Build history of the part. All positions in model axes, mm. A direction names the side the tool comes from. Coordinates: 2 decimals unless noted, no trailing zeros. Order: outer loops, then holes, each group sorted by start corner. A loop starts at its lowest first (then second) coordinate and runs counter-clockwise, first axis right, second up. Notation, with made-up numbers: (44, 35.25) - (96, 35.25) arc R23 cw to (96, 59.25) - close; hole circle Ø1 at (74.5, 42). An arc over 180 degrees is marked (long way). Write each question's results on one line, items separated by ' | '.
from build123d import *

# Parameters (mm, degrees)
BOSS_EXTRUDE1_DEPTH = 50
SKETCH2_R           = 2.8
CUT_EXTRUDE1_DEPTH  = 53.73966846


with BuildPart() as part:
    # Sketch1 → Boss-Extrude1 (new body)
    with BuildSketch(Plane.XY):
        with BuildLine():
            Line((-10.618380291, 0), (10.618380291, 0))
            Line((10.618380291, 0), (10.618380291, 6))
            ThreePointArc((10.618380291, 6), (7.305893165, 8.590308493), (3.395577503, 10.136820848))
            Line((3.395577503, 10.136820848), (3.395577503, 10.989327513))
            ThreePointArc((3.395577503, 10.989327513), (2.809791065, 12.403541075), (1.395577503, 12.989327513))
            Line((1.395577503, 12.989327513), (-1.395577503, 12.989327513))
            ThreePointArc((-1.395577503, 12.989327513), (-2.809791065, 12.403541075), (-3.395577503, 10.989327513))
            Line((-3.395577503, 10.989327513), (-3.395577503, 10.136820848))
            ThreePointArc((-3.395577503, 10.136820848), (-7.305893165, 8.590308493), (-10.618380291, 6))
            Line((-10.618380291, 6), (-10.618380291, 0))
        make_face()
    extrude(amount=-BOSS_EXTRUDE1_DEPTH)

    # Sketch2 → Cut-Extrude1 (cut, through all)
    with BuildSketch(Plane.XY):
        with Locations((-4, 4.84)):
            Circle(SKETCH2_R)
        with Locations((4, 4.84)):
            Circle(SKETCH2_R)
    extrude(amount=-CUT_EXTRUDE1_DEPTH, mode=Mode.SUBTRACT)


solid = part.part
1. Band-saw the part on C-C on x = -4. Give the cut face in (y, z), then the cut area to 3 significant figures.
Solved:
outline: (0, -50) - (2.04, -50) - (2.04, 0) - (0, 0) - close; (7.64, -50) - (9.98, -50) - (9.98, 0) - (7.64, 0) - close | area: 219 mm2
2. Band-saw the part on D-D on x = 5.5. Give the cut face in (y, z), then the cut area to 3 significant figures.
Solved:
outline: (0, -50) - (2.48, -50) - (2.48, 0) - (0, 0) - close; (7.2, -50) - (9.47, -50) - (9.47, 0) - (7.2, 0) - close | area: 237 mm2
3. Band-saw the part on A-A on y = 4.84. Give the cut face in (x, z), then the cut area to 3 significant figures.
Solved:
outline: (-10.62, -50) - (-6.8, -50) - (-6.8, 0) - (-10.62, 0) - close; (-1.2, -50) - (1.2, -50) - (1.2, 0) - (-1.2, 0) - close; (6.8, -50) - (10.62, -50) - (10.62, 0) - (6.8, 0) - close | area: 502 mm2
4. Probe line 1 (X direction, y = 2.5, z = -33.5); line 2 (X direction, y = 7.25, z = -6.5); line 3 (X direction, y = 11, z = -29). List the from-to ranges inside material, lowest first.
Solved:
line 1: x = -10.62 to -5.54, -2.46 to 2.46, 5.54 to 10.62 | line 2: x = -9.26 to -5.43, -2.57 to 2.57, 5.43 to 9.26 | line 3: x = -3.4 to 3.4
5. Drop flat-ended pins along their axis: pin 1 Ø0.7 at (y, z) = (11, -17) entering from +X; pin 2 Ø1.5 at (x, y) = (-3, 5.5) entering from +Z; pin 3 Ø2 at (x, z) = (6, -12) entering from +Y. Give the stop position or say it passes through.
Solved:
pin 1: stops at x = 3.4 | pin 2: passes through | pin 3: stops at y = 9.66
6. Two-plate mould, pull along Y, no slides. Class faces 1 (the face through (-10.618, 3, -25)), 2 (the face through (0, 12.989, -25)), 3 (the face through (3.635, 7.616, -24.65)): +Y half, -Y half, draft (parallel to the pull), parting line (faces both ways), or undercut.
Solved:
face 1: draft | face 2: +Y half | face 3: undercut
7. Band-saw the part on B-B on z = -24.5. Give the cut face in (x, y), then the cut area to 3 significant figures.
Solved:
outline: (-10.62, 0) - (10.62, 0) - (10.62, 6) arc R14.7 ccw to (3.4, 10.14) - (3.4, 10.99) arc R2 ccw to (1.4, 12.99) - (-1.4, 12.99) arc R2 ccw to (-3.4, 10.99) - (-3.4, 10.14) arc R14.7 ccw to (-10.62, 6) - close; hole circle Ø5.6 at (-4, 4.84); hole circle Ø5.6 at (4, 4.84) | area: 160 mm2
8. Tool access for faces 4 (the face through (-3.396, 10.6, -24.6)), 5 (the face through (-2.49, 7.2, -24.65)), 6 (the face through (3.396, 10.6, -24.6)): list every direction of +Z, -Z, +X, -X, +Y, -Y with a clear straight run to the whole face (end or side of a thin tool).
Solved:
face 4: +Z, -Z, -X, +Y | face 5: +Z, -Z | face 6: +Z, -Z, +X, +Y
